Here's how the part is built. I have some questions about the finished solid (model axes, mm). Face numbers are marked on the shaded views. A direction names the side the tool comes from. Give positions to 0.01 mm unless a question says otherwise; leave off trailing zeros. Write each loop counter-clockwise with the first axis right and the second up, starting at its lowest first coordinate (ties: lowest second). Pieces come first, ordered by that corner, then holes. Notation, with made-up numbers: (51, -16) -> (105, -16) arc R28 ccw to (105, 19) -> close; hole circle Ø9 at (81, 43). An arc over 180 degrees is marked (long way). Use CSV: the item, a comma, the result in double quotes. Start each with the question number.
(1) Which directions (+Z, -Z, +X, -X, +Y, -Y) give clear straight access to the entire face, cutting with the end or side of a thin tool? Please do the marked faces 4 and 5.
(2) If we mould it in two halves opening along Z, with no side actions, what happens to the marked faces 1, 2 and 3? For each: pulls with the +Z half, pulls with the -Z half, needs draft (parallel to the pull), parting line crosses it, or undercut.
(3) Suppose I cut it at A-A on x = -38.1. List the corners of the cut face in (y, z) for me (3 decimals).
(4) Suppose I cut it at D-D on z = 71.5. List the corners of the cut face in (x, y) for me (3 decimals).
(5) Suppose I cut it at C-C on y = -20.32. Give the number of separate pieces and of enclosed holes in the cut face, plus the area to 3 significant figures.
(6) Suppose I cut it at B-B on y = 5. List the corners of the cut face in (x, z) for me, plus the area to 3 significant figures.
(7) For pin 1 Ø5.5 at (y, z) = (-19, 87) entering from -X; pin 2 Ø6 at (x, y) = (39, -3) entering from -Z; pin 3 Ø4 at (x, y) = (-17.2, -10.41) entering from -Z; pin 4 Ø2.5 at (y, z) = (-17.5, 114.5) entering from +X, each with a flat end and sliding along its axis, tell me the tip position at first contact or that it passes through.
(8) I need wall thicknesses on L1, parallel to Y at x = -38.1, z = 114.5 (3 decimals); L2, parallel to Z at x = -41, y = -10.5; L3, parallel to Y at x = 26.5, z = 111. Which ranges of each line are inside material? Lowest first, please. Write a range as [from, to].
from build123d import *
from build123d.topology import SkipClean

# Parameters (mm, degrees)
SKETCH2_R                       = 7.9756
BOSS_EXTRUDE1_DEPTH             = 7.9502
SKETCH3_W                       = 107.95
SKETCH3_H                       = 6.35
BOSS_EXTRUDE2_DEPTH             = 101.6
SKETCH4_R                       = 7.9756
BOSS_EXTRUDE3_DEPTH             = 7.9502
SKETCH5_W                       = 117.5004
SKETCH5_H                       = 6.35
BOSS_EXTRUDE4_DEPTH             = 6.35
SKETCH6_W                       = 33.463288309
SKETCH6_H                       = 6.35
BOSS_EXTRUDE5_DEPTH             = 19.05
BOSS_EXTRUDE6_START             = -33.463288
BOSS_EXTRUDE6_DEPTH             = 33.463288
BOSS_EXTRUDE8_DEPTH             = 8.83271
M4X0_7_TAPPED_HOLE1_D           = 3.3
M4X0_7_TAPPED_HOLE1_CSINK_D     = 4.05
M4X0_7_TAPPED_HOLE1_CSINK_ANGLE = 90
CUT_EXTRUDE1_REACH              = 124.266
SKETCH15_R                      = 1.651
CUT_EXTRUDE2_REACH              = 128.428
SKETCH18_R                      = 1.651
SKETCH19_W                      = 7.62
SKETCH19_H                      = 12.7
BOSS_EXTRUDE9_DEPTH             = 31.75


with BuildPart() as part:
    # Sketch2 → Boss-Extrude1 (new body)
    with BuildSketch(Plane.XY):
        with BuildLine():
            Line((-22.225, -25.4), (-22.225, 0))
            ThreePointArc((-22.225, 0), (-38.1, 15.875), (-53.975, 0))
            Line((-53.975, 0), (-53.975, -31.75))
            Line((-53.975, -31.75), (53.975, -31.75))
            Line((53.975, -31.75), (53.975, -25.4))
            Line((53.975, -25.4), (22.225, -25.4))
            Line((22.225, -25.4), (-22.225, -25.4))
        make_face()
        with Locations((-38.1, 0)):
            Circle(SKETCH2_R, mode=Mode.SUBTRACT)
    extrude(amount=BOSS_EXTRUDE1_DEPTH)

    # Sketch3 → Boss-Extrude2 (add)
    with BuildSketch(Plane.XY.offset(7.9502)):
        with Locations((0, -28.575)):
            Rectangle(SKETCH3_W, SKETCH3_H)
    extrude(amount=BOSS_EXTRUDE2_DEPTH)

    # Sketch4 → Boss-Extrude3 (add)
    with BuildSketch(Plane.XY.offset(109.5502)):
        with BuildLine():
            Line((-53.975, 0), (-53.975, -31.75))
            Line((-53.975, -31.75), (53.975, -31.75))
            Line((53.975, -31.75), (53.975, -25.4))
            Line((53.975, -25.4), (-22.225, -25.4))
            Line((-22.225, -25.4), (-22.225, 0))
            ThreePointArc((-22.225, 0), (-38.1, 15.875), (-53.975, 0))
        make_face()
        with Locations((-38.1, 0)):
            Circle(SKETCH4_R, mode=Mode.SUBTRACT)
    extrude(amount=BOSS_EXTRUDE3_DEPTH)

    # Sketch5 → Boss-Extrude4 (add)
    with BuildSketch(Plane(origin=(53.975, 0, 0), x_dir=(0, 0, -1), z_dir=(1, 0, 0))):
        with Locations((-58.7502, -28.575)):
            Rectangle(SKETCH5_W, SKETCH5_H)
    extrude(amount=BOSS_EXTRUDE4_DEPTH)

    # Sketch6 → Boss-Extrude5 (add)
    with BuildSketch(Plane(origin=(0, -25.4, 0), x_dir=(1, 0, 0), z_dir=(0, 1, 0))):
        with Locations((43.593355845, -98.3234)):
            Rectangle(SKETCH6_W, SKETCH6_H)
        Polygon((-13.392288309, -112.8252), (-13.392288309, -107.418332231), (-16.329801264, -106.4752), (-21.012288309, -106.4752), (-21.012288309, -109.5502), (-22.225, -109.5502), (-22.225, -112.8252), align=None)
    extrude(amount=BOSS_EXTRUDE5_DEPTH)

    # Sketch8 → Boss-Extrude6 (add)
    with SkipClean():  # the faces are left unmerged after this step: merging them gives an invalid solid
        with BuildSketch(Plane(origin=(60.325, 0, 0), x_dir=(0, 0, -1), z_dir=(1, 0, 0)).offset(BOSS_EXTRUDE6_START)):
            Polygon((-95.1484, -6.35), (-76.0984, -25.4), (-95.1484, -25.4), align=None)
        extrude(amount=BOSS_EXTRUDE6_DEPTH)

    # Sketch10 → Boss-Extrude8 (add)
    with SkipClean():  # the faces are left unmerged after this step: merging them gives an invalid solid
        with BuildSketch(Plane(origin=(-22.225, 0, 0), x_dir=(0, 0, -1), z_dir=(1, 0, 0))):
            Polygon((-112.8252, -6.35), (-117.5004, -25.4), (-112.8252, -25.4), align=None)
        extrude(amount=BOSS_EXTRUDE8_DEPTH)

    # M4x0.7 Tapped Hole1 (through all)
    with Locations(Plane(origin=(0, -25.4, 0), x_dir=(1, 0, 0), z_dir=(0, 1, 0))):
        with Locations((6.876306211, -48.0502), (6.876306211, -67.1002), (-31.223693789, -67.1002), (-31.223693789, -48.0502)):
            CounterSinkHole(M4X0_7_TAPPED_HOLE1_D / 2, M4X0_7_TAPPED_HOLE1_CSINK_D / 2, counter_sink_angle=M4X0_7_TAPPED_HOLE1_CSINK_ANGLE)

    # Cut-Extrude1: up to this plane
    with SkipClean():  # the faces are left unmerged after this step: merging them gives an invalid solid
        cut_extrude1_end = Plane(origin=(26.861711691, -6.35, 95.1484), z_dir=(0, 0.7071067811865517, -0.7071067811865435))
        # Sketch15 → Cut-Extrude1 (cut, up to the surface)
        with BuildSketch(Plane.XY.offset(101.4984), mode=Mode.PRIVATE) as cut_extrude1_sk1:
            with Locations((30.925711691, -10.414)):
                Circle(SKETCH15_R)
        cut_extrude1_tool1 = split(extrude(cut_extrude1_sk1.sketch, amount=-CUT_EXTRUDE1_REACH, mode=Mode.PRIVATE), bisect_by=cut_extrude1_end, keep=Keep.BOTH, mode=Mode.PRIVATE)
        add(cut_extrude1_tool1.solids().sort_by_distance((30.925712, -10.414, 101.4984))[0], mode=Mode.SUBTRACT)
        # Sketch15 → Cut-Extrude1 (cut, up to the surface)
        with BuildSketch(Plane.XY.offset(101.4984), mode=Mode.PRIVATE) as cut_extrude1_sk2:
            with Locations((30.925711691, -20.32)):
                Circle(SKETCH15_R)
        cut_extrude1_tool2 = split(extrude(cut_extrude1_sk2.sketch, amount=-CUT_EXTRUDE1_REACH, mode=Mode.PRIVATE), bisect_by=cut_extrude1_end, keep=Keep.BOTH, mode=Mode.PRIVATE)
        add(cut_extrude1_tool2.solids().sort_by_distance((30.925712, -20.32, 101.4984))[0], mode=Mode.SUBTRACT)

    # Cut-Extrude2: up to this plane
    with SkipClean():  # the faces are left unmerged after this step: merging them gives an invalid solid
        cut_extrude2_end = Plane(origin=(-13.392288309, -6.35, 112.8252), z_dir=(0, -0.23834455727061551, -0.9711806587960216))
        # Sketch18 → Cut-Extrude2 (cut, up to the surface)
        with BuildSketch(Plane(origin=(0, 0, 106.4752), x_dir=(-1, 0, 0), z_dir=(0, 0, -1)), mode=Mode.PRIVATE) as cut_extrude2_sk1:
            with Locations(Location((17.202288309, -10.414, 0), (0, 0, 90))):
                Circle(SKETCH18_R)
        cut_extrude2_tool1 = split(extrude(cut_extrude2_sk1.sketch, amount=-CUT_EXTRUDE2_REACH, mode=Mode.PRIVATE), bisect_by=cut_extrude2_end, keep=Keep.BOTH, mode=Mode.PRIVATE)
        add(cut_extrude2_tool1.solids().sort_by_distance((-17.202288, -10.414, 106.4752))[0], mode=Mode.SUBTRACT)
        # Sketch18 → Cut-Extrude2 (cut, up to the surface)
        with BuildSketch(Plane(origin=(0, 0, 106.4752), x_dir=(-1, 0, 0), z_dir=(0, 0, -1)), mode=Mode.PRIVATE) as cut_extrude2_sk2:
            with Locations(Location((17.202288309, -20.32, 0), (0, 0, 90))):
                Circle(SKETCH18_R)
        cut_extrude2_tool2 = split(extrude(cut_extrude2_sk2.sketch, amount=-CUT_EXTRUDE2_REACH, mode=Mode.PRIVATE), bisect_by=cut_extrude2_end, keep=Keep.BOTH, mode=Mode.PRIVATE)
        add(cut_extrude2_tool2.solids().sort_by_distance((-17.202288, -20.32, 106.4752))[0], mode=Mode.SUBTRACT)

    # Sketch19 → Boss-Extrude9 (add)
    with SkipClean():  # the faces are left unmerged after this step: merging them gives an invalid solid
        with BuildSketch(Plane.ZY.offset(53.975)):
            with Locations((11.7602, -19.05)):
                Rectangle(SKETCH19_W, SKETCH19_H)
            with Locations((105.7402, -19.05)):
                Rectangle(SKETCH19_W, SKETCH19_H)
        extrude(amount=-BOSS_EXTRUDE9_DEPTH)


solid = part.part
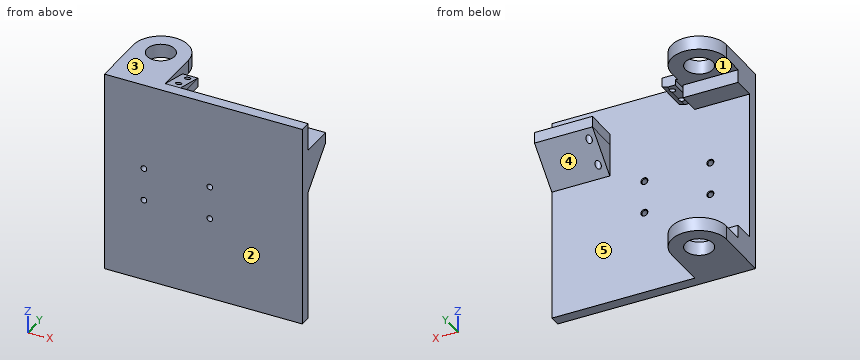
Geometry says:
1,face 4,"-Z, +X, -X, +Y"
1,face 5,"+Y"
2,face 1,"undercut"
2,face 2,"needs draft"
2,face 3,"pulls with the +Z half"
3,outline,"(-31.75, 0) -> (-7.976, 0) -> (-7.976, 7.95) -> (-12.7, 7.95) -> (-12.7, 15.57) -> (-25.4, 15.57) -> (-25.4, 101.93) -> (-12.7, 101.93) -> (-12.7, 109.55) -> (-7.976, 109.55) -> (-7.976, 117.5) -> (-31.75, 117.5) -> close; (7.976, 0) -> (15.875, 0) -> (15.875, 7.95) -> (7.976, 7.95) -> close; (7.976, 109.55) -> (15.875, 109.55) -> (15.875, 117.5) -> (7.976, 117.5) -> close"
4,outline,"(-53.975, -31.75) -> (60.325, -31.75) -> (60.325, -25.4) -> (-53.975, -25.4) -> close"
5,separate pieces,"5"
5,enclosed holes,"0"
5,area,"1,650 mm²"
6,outline,"(-53.17, 0) -> (-44.31, 0) -> (-44.31, 7.95) -> (-53.17, 7.95) -> close; (-53.17, 109.55) -> (-44.31, 109.55) -> (-44.31, 117.5) -> (-53.17, 117.5) -> close; (-31.89, 0) -> (-23.03, 0) -> (-23.03, 7.95) -> (-31.89, 7.95) -> close; (-31.89, 109.55) -> (-23.03, 109.55) -> (-23.03, 117.5) -> (-31.89, 117.5) -> close"
6,area,"282 mm²"
7,pin 1,"x = 26.86"
7,pin 2,"through"
7,pin 3,"z = 106.48"
7,pin 4,"x = -13.39"
8,L1,"[-31.75, -7.976], [7.976, 15.875]"
8,L2,"[0, 7.95], [109.55, 117.5]"
8,L3,"[-31.75, -25.4]"
